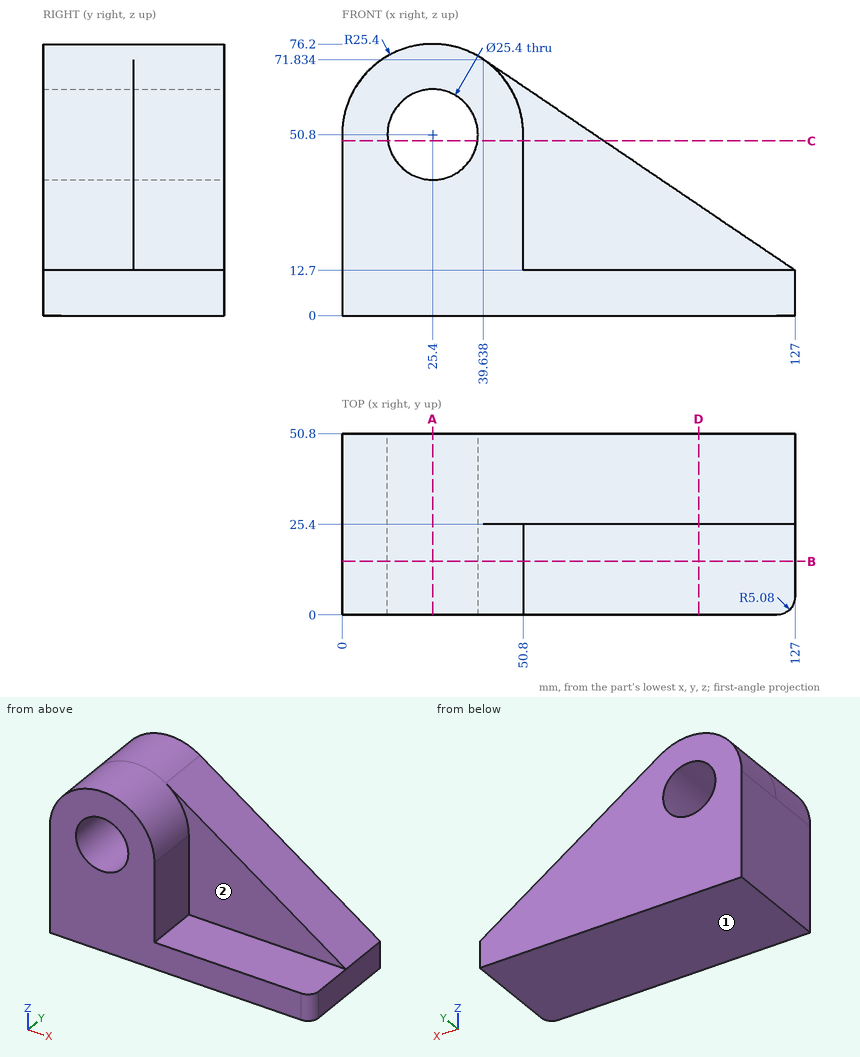
Check sheet for the drawn part. Datum: minimum x, y, z corner. Units: mm. A direction names the side the tool comes from. Round coordinates to 2 decimals unless told otherwise and drop trailing zeros. Loops run counter-clockwise (first coordinate to the right, second up) from the corner with the lowest first, then second, coordinate; pieces in that order, holes last. Notation, with made-up numbers: (73.25, 37) - (114.25, 37) arc R18 cw to (114.25, 56) - close; hole circle Ø7 at (75.25, 0.25). An arc over 180 degrees is marked (long way). Use one line per item in the form item = value.
1. Section check C-C on z = 49. Record the cut outline in (x, y), and give its area (3 significant figures).
A:
outline = (0, 0) - (12.83, 0) - (12.83, 50.8) - (0, 50.8) - close; (37.97, 0) - (50.8, 0) - (50.8, 25.4) - (73.37, 25.4) - (73.37, 50.8) - (37.97, 50.8) - close
area = 1,880 mm²
2. Gauge pin test, flat ends, axial feed: pin 1 Ø4 at (y, z) = (7, 18.5) entering from +X; pin 2 Ø12.5 at (x, y) = (96.5, 19) entering from +Z; pin 3 Ø12 at (x, y) = (108, 31) entering from +Z. Record the tip position at first contact, or that the pin passes through.
A:
pin_1 = 50.8
pin_2 = 12.7
pin_3 = 29.62
3. Access from +Z, -Z, +X, -X, +Y, -Y to the whole of each face (thin tool, end or side, straight path). Record for the marked faces 1 and 2.
A:
face_1 = -Z, +X, -X, +Y, -Y
face_2 = +Z, +X, -Y
4. Scan lines: probe 1 along X at (y, z) = (13, 50) (1 decimal); probe 2 along Z at (x, y) = (25.4, 24.5); probe 3 along Z at (x, y) = (83.5, 3.5). Record each from-to range of solid material in increasing order.
A:
probe_1 = 0 to 12.7, 38.1 to 50.8
probe_2 = 0 to 38.1, 63.5 to 76.2
probe_3 = 0 to 12.7
5. Section check A-A on x = 25.4. Record the cut outline in (y, z).
A:
outline = (0, 0) - (50.8, 0) - (50.8, 38.1) - (0, 38.1) - close; (0, 63.5) - (50.8, 63.5) - (50.8, 76.2) - (0, 76.2) - close
6. Section check D-D on x = 100. Record the cut outline in (y, z).
A:
outline = (0, 0) - (50.8, 0) - (50.8, 30.98) - (25.4, 30.98) - (25.4, 12.7) - (0, 12.7) - close
7. Section check B-B on y = 15. Record the cut outline in (x, z), and give its area (4 significant figures).
A:
outline = (0, 0) - (127, 0) - (127, 12.7) - (50.8, 12.7) - (50.8, 50.8) arc R25.4 ccw to (0, 50.8) - close; hole circle Ø25.4 at (25.4, 50.8)
area = 4,055 mm²
